Verification items for this drawing (mm, ordinates from the low corner). A direction names the side the tool comes from. Coordinates: 2 decimals unless noted, no trailing zeros. Order: outer loops, then holes, each group sorted by start corner. A loop starts at its lowest first (then second) coordinate and runs counter-clockwise, first axis right, second up. Notation, with made-up numbers: M 50.5,-26.5 L 54.5,-26.5 A31 ccw 54.5,1.5 Z; hole C -8.5,43 d10. An arc over 180 degrees is marked long. Answer as a JSON object with one key per item and string values. Group by question number.
(1) Cross-section at C-C (y = 1.75). Enter the section's corners in (x, z), plus the area to 3 significant figures.
(2) Cross-section at B-B (z = 8). Enter the section's corners in (x, y), plus the area to 3 significant figures.
(3) Cross-section at A-A (x = 11.25). Enter the section's corners in (y, z).
(4) Material ranges on line 1 (Z direction, x = 11.25, y = 2.65); line 2 (Y direction, x = 6, z = 18.5), recorded low to high.
(5) Gauge pin test, flat ends, axial feed: pin 1 Ø1.5 at (y, z) = (6.5, 14.5) entering from +X; pin 2 Ø9 at (x, z) = (14.5, 7.5) entering from +Y; pin 3 Ø5 at (y, z) = (5.5, 7.5) entering from -X; pin 4 Ø11 at (x, z) = (11.25, 11.25) entering from +Y. Record the tip position at first contact, or that the pin passes through.
(6) Access from +Z, -Z, +X, -X, +Y, -Y to the whole of each face (thin tool, end or side, straight path). Record for the marked faces 1, 2 and 3.
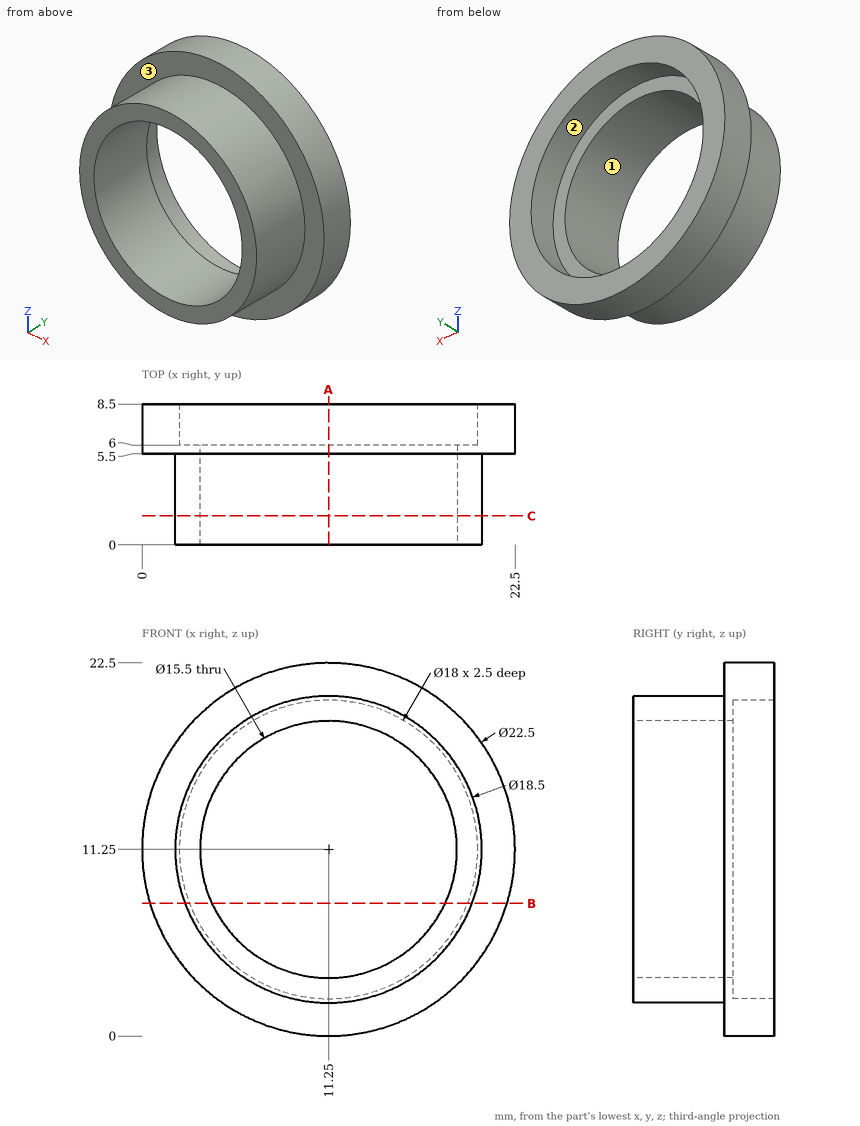
Taken from the geometry:
{
 "1": {"outline": "C 11.25,11.25 d18.5; hole C 11.25,11.25 d15.5", "area": "80.1 mm²"},
 "2": {"outline": "M 0.48,5.5 L 2.59,5.5 L 2.59,0 L 4.21,0 L 4.21,6 L 2.86,6 L 2.86,8.5 L 0.48,8.5 Z; M 18.29,0 L 19.91,0 L 19.91,5.5 L 22.02,5.5 L 22.02,8.5 L 19.64,8.5 L 19.64,6 L 18.29,6 Z", "area": "33.5 mm²"},
 "3": {"outline": "M 0,2 L 5.5,2 L 5.5,0 L 8.5,0 L 8.5,2.25 L 6,2.25 L 6,3.5 L 0,3.5 Z; M 0,19 L 6,19 L 6,20.25 L 8.5,20.25 L 8.5,22.5 L 5.5,22.5 L 5.5,20.5 L 0,20.5 Z"},
 "4": {"line 1": "z = 2 to 3.5, 19 to 20.5", "line 2": "y = 0 to 6"},
 "5": {"pin 1": "stops at x = 22.22", "pin 2": "stops at y = 8.5", "pin 3": "stops at x = 0.07", "pin 4": "passes through"},
 "6": {"face 1": "+Y, -Y", "face 2": "+Y", "face 3": "-Y"}
}
